Geometry check sheet. Reference: the model listing, model coordinates, mm. A direction names the side the tool comes from. Give positions to 0.01 mm unless a question says otherwise; leave off trailing zeros. Write each loop counter-clockwise with the first axis right and the second up, starting at its lowest first coordinate (ties: lowest second). Pieces come first, ordered by that corner, then holes. Notation, with made-up numbers: (64, -10) - (97, -10) arc R24 ccw to (97, 20) - close; hole circle Ø2 at (43, 2). An arc over 180 degrees is marked (long way). Use a Markdown table: item, result.
```python
from build123d import *

# Parameters (mm, degrees)
SKETCH1_R           = 5
SKETCH1_R_2         = 2.83
SKETCH1_R_3         = 3.25
SKETCH1_W           = 8.7
SKETCH1_H           = 3.4
BOSS_EXTRUDE1_DEPTH = 4
BOSS_EXTRUDE2_DEPTH = 4


with BuildPart() as part:
    # Sketch1 → Boss-Extrude1 (new body)
    with BuildSketch(Plane.XY):
        Polygon((49, 30), (56.5, 30), (56.5, 25), (64.5, 25), (64.5, 17), (56.5, 17), (56.5, 13), (49.7, 13), (49.7, -13), (56.5, -13), (56.5, -17), (64.5, -17), (64.5, -25), (56.5, -25), (56.5, -30), (49, -30), (-79, -30), (-79, 30), align=None)
        with Locations((-46, 0)):
            Circle(SKETCH1_R, mode=Mode.SUBTRACT)
        with Locations((25, -24)):
            Circle(SKETCH1_R_2, mode=Mode.SUBTRACT)
        with Locations((-12.5, 24.5)):
            Circle(SKETCH1_R_3, mode=Mode.SUBTRACT)
        with Locations((30.35, -13.3)):
            Rectangle(SKETCH1_W, SKETCH1_H, mode=Mode.SUBTRACT)
    extrude(amount=BOSS_EXTRUDE1_DEPTH)

    # Sketch2 → Boss-Extrude2 (add)
    with BuildSketch(Plane.XY):
        Polygon((-79, 30), (56.5, 30), (56.5, 55), (41.5, 55), (27.357864376, 40.857864376), (-49.857864376, 40.857864376), (-64, 55), (-79, 55), align=None)
    extrude(amount=BOSS_EXTRUDE2_DEPTH)


solid = part.part
```
1) Section check A-A on y = 44. Record the boundary of the cut face in (x, z), then the cut area to 3 significant figures.
Working result:
| item | result |
|---|---|
| outline | (-79, 0) - (-53, 0) - (-53, 4) - (-79, 4) - close; (30.5, 0) - (56.5, 0) - (56.5, 4) - (30.5, 4) - close |
| area | 208 mm² |
2) Section check C-C on z = 3.2. Record the boundary of the cut face in (x, y), then the cut area to 3 significant figures.
Working result:
| item | result |
|---|---|
| outline | (-79, -30) - (56.5, -30) - (56.5, -25) - (64.5, -25) - (64.5, -17) - (56.5, -17) - (56.5, -13) - (49.7, -13) - (49.7, 13) - (56.5, 13) - (56.5, 17) - (64.5, 17) - (64.5, 25) - (56.5, 25) - (56.5, 55) - (41.5, 55) - (27.36, 40.86) - (-49.86, 40.86) - (-64, 55) - (-79, 55) - close; hole circle Ø10 at (-46, 0); hole circle Ø6.5 at (-12.5, 24.5); hole circle Ø5.66 at (25, -24); hole (26, -15) - (34.7, -15) - (34.7, -11.6) - (26, -11.6) - close |
| area | 10,000 mm² |
3) Set-up check for faces 4 (the flat face through (34.5, 48, 2)), 5 (the flat face through (30, -15, 2)), 6 (the flat face through (56.5, 15, 2)), 7 (the flat face through (61, -25, 2)): record each of +Z, -Z, +X, -X, +Y, -Y from which the full face is reachable in a straight line by a thin tool's end or side.
Working result:
| item | result |
|---|---|
| face 4 | +Z, -Z, +Y |
| face 5 | +Z, -Z |
| face 6 | +Z, -Z, +X |
| face 7 | +Z, -Z, +X, -Y |
4) Material ranges on L1, parallel to Y at x = 25, z = 2.1; L2, parallel to Y at x = -46, z = 1.05; L3, parallel to X at y = 41, z = 1.9, recorded low to high. Write a range as from..to.
Working result:
| item | result |
|---|---|
| L1 | y = -30..-26.83, -21.17..40.86 |
| L2 | y = -30..-5, 5..40.86 |
| L3 | x = -79..-50, 27.5..56.5 |
5) Section check B-B on x = 51.5. Record the boundary of the cut face in (y, z).
Working result:
| item | result |
|---|---|
| outline | (-30, 0) - (-13, 0) - (-13, 4) - (-30, 4) - close; (13, 0) - (55, 0) - (55, 4) - (13, 4) - close |
6) Section check D-D on y = 35. Record the boundary of the cut face in (x, z), then the cut area to 3 significant figures.
Working result:
| item | result |
|---|---|
| outline | (-79, 0) - (56.5, 0) - (56.5, 4) - (-79, 4) - close |
| area | 542 mm² |
7) Mould release check, pull along Y, two halves, no side actions. Record for faces 1 (the flat face through (56.5, 40, 2)), 2 (the flat face through (49, 55, 2)), 3 (the flat face through (30, -11.6, 2)): pulls with the +Y half, pulls with the -Y half, needs draft (parallel to the pull), parting line crosses it, or undercut.
Working result:
| item | result |
|---|---|
| face 1 | needs draft |
| face 2 | pulls with the +Y half |
| face 3 | undercut |
8) Depth check by flat-ended pin: P1, Ø1.2, axis at x = 62, z = 3, coming from the -Y side; P2, Ø1, axis at y = -14, z = 1, coming from the +X side. Enter the tip coordinate at first touch or a pass-through.
Working result:
| item | result |
|---|---|
| P1 | stops at y = -25 |
| P2 | stops at x = 56.5 |
